from build123d import *

# Parameters (mm, degrees)
BOSS_EXTRUDE1_DEPTH = 100
BOSS_EXTRUDE3_DEPTH = 15


with BuildPart() as part:
    # Sketch3 → Boss-Extrude1 (new body)
    with BuildSketch(Plane(origin=(0, 0, 0), x_dir=(1, 0, 0), z_dir=(0, 1, 0))):
        with BuildLine():
            Line((123.743686708, 123.743686708), (30.045678616, 26.405628121))
            ThreePointArc((30.045678616, 26.405628121), (37.863583917, 12.897635944), (39.917101801, -2.573904389))
            Line((39.917101801, -2.573904389), (175, 0))
            ThreePointArc((175, 0), (161.678918189, 66.969600664), (123.743686708, 123.743686708))
        make_face()
        with BuildLine():
            Line((36.672129032, 26.079780525), (123.758669753, 116.549524499))
            ThreePointArc((123.758669753, 116.549524499), (157.096506553, 64.966819445), (169.929243976, 4.904288086))
            Line((169.929243976, 4.904288086), (44.929243976, 2.52250584))
            ThreePointArc((44.929243976, 2.52250584), (42.466837849, 14.885149752), (36.672129032, 26.079780525))
        make_face(mode=Mode.SUBTRACT)
    extrude(amount=BOSS_EXTRUDE1_DEPTH)

    # Sketch5 → Boss-Extrude3 (add)
    with BuildSketch(Plane(origin=(0, 0, 0), x_dir=(1, 0, 0), z_dir=(0, 1, 0))):
        with BuildLine():
            Line((39.917101801, -2.573904389), (175, 0))
            ThreePointArc((175, 0), (161.678918189, 66.969600664), (123.743686708, 123.743686708))
            Line((123.743686708, 123.743686708), (30.045678616, 26.405628121))
            ThreePointArc((30.045678616, 26.405628121), (37.863583917, 12.897635944), (39.917101801, -2.573904389))
        make_face()
    extrude(amount=BOSS_EXTRUDE3_DEPTH)


solid = part.part
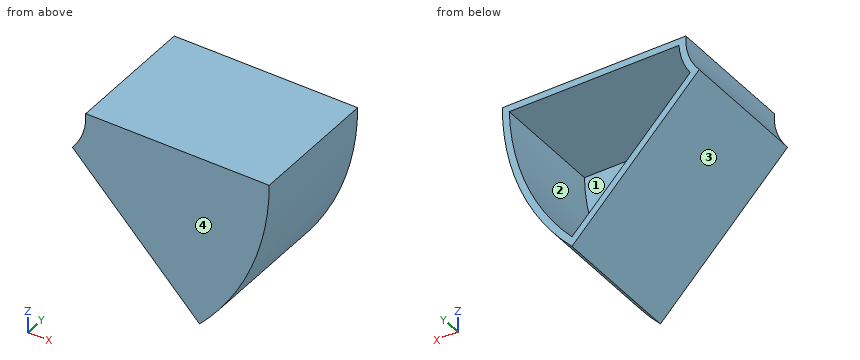
Here's how the part is built. I have some questions about the finished solid (model axes, mm). Face numbers are marked on the shaded views. Round coordinates to 2 decimals unless told otherwise and drop trailing zeros. Loops run counter-clockwise (first coordinate to the right, second up) from the corner with the lowest first, then second, coordinate; pieces in that order, holes last. Notation, with made-up numbers: M 74.5,53 L 133.5,53 A22 ccw 133.5,85 Z; hole C 89,27 d8. An arc over 180 degrees is marked long. Write each question's results on one line, items separated by ' | '. Start each with the question number.
(1) I want a section at A-A (y = 53). Please give me the cut outline in (x, z).
(2) I want a section at D-D (y = 8). Please give me the cut outline in (x, z), then the cut area to 3 significant figures.
(3) I want a section at B-B (z = -55). Please give me the cut outline in (x, y), then the cut area to 3 significant figures.
(4) Will these pins go through, and if not, where does the flat tip stop? P1, Ø5, axis at x = 58, z = -35, coming from the +Y side; P2, Ø6, axis at x = 48.5, y = 64, coming from the -Z side; P3, Ø5, axis at y = 48, z = -29, coming from the -X side.
(5) If I drill on probe 1 along Z at (x, y) = (65.5, 31); probe 2 along X at (y, z) = (51, -14); probe 3 along Z at (x, y) = (102.5, 65), over which ranges is the centre line in solid material (lowest first)? Write a range as from..to.
(6) I want a section at C-C (x = 111). Please give me the cut outline in (y, z), then the cut area to 3 significant figures.
(7) Thinking about a two-plate mould opening in Z: for the marked faces 1, 2, 3 and 4, which applies, pulls with the +Z half, pulls with the -Z half, needs draft (parallel to the pull), parting line crosses it, or undercut?
Solved:
1) outline: M 30.05,-26.41 L 123.74,-123.74 A175 ccw 175,0 L 39.92,2.57 A40 cw Z; hole M 36.67,-26.08 L 123.76,-116.55 A170 ccw 169.93,-4.9 L 44.93,-2.52 A45 cw Z
2) outline: M 30.05,-26.41 L 123.74,-123.74 A175 ccw 175,0 L 39.92,2.57 A40 cw Z | area: 11,400 mm²
3) outline: M 57.57,0 L 166.13,0 L 166.13,100 L 160.86,100 L 160.86,15 L 64.51,15 L 64.51,100 L 57.57,100 Z | area: 2,670 mm²
4) P1: stops at y = 15 | P2: stops at z = -48.69 | P3: stops at x = 30.14
5) probe 1: z = -63.24..-56.03, -2.91..2.09 | probe 2: x = 37.47..42.77, 169.42..174.44 | probe 3: z = -101.67..-94.46, -3.62..1.38
6) outline: M 0,-110.5 L 100,-110.5 L 100,-103.3 L 15,-103.3 L 15,-3.78 L 100,-3.78 L 100,1.22 L 0,1.22 Z | area: 2,710 mm²
7) face 1: undercut | face 2: undercut | face 3: pulls with the -Z half | face 4: needs draft
